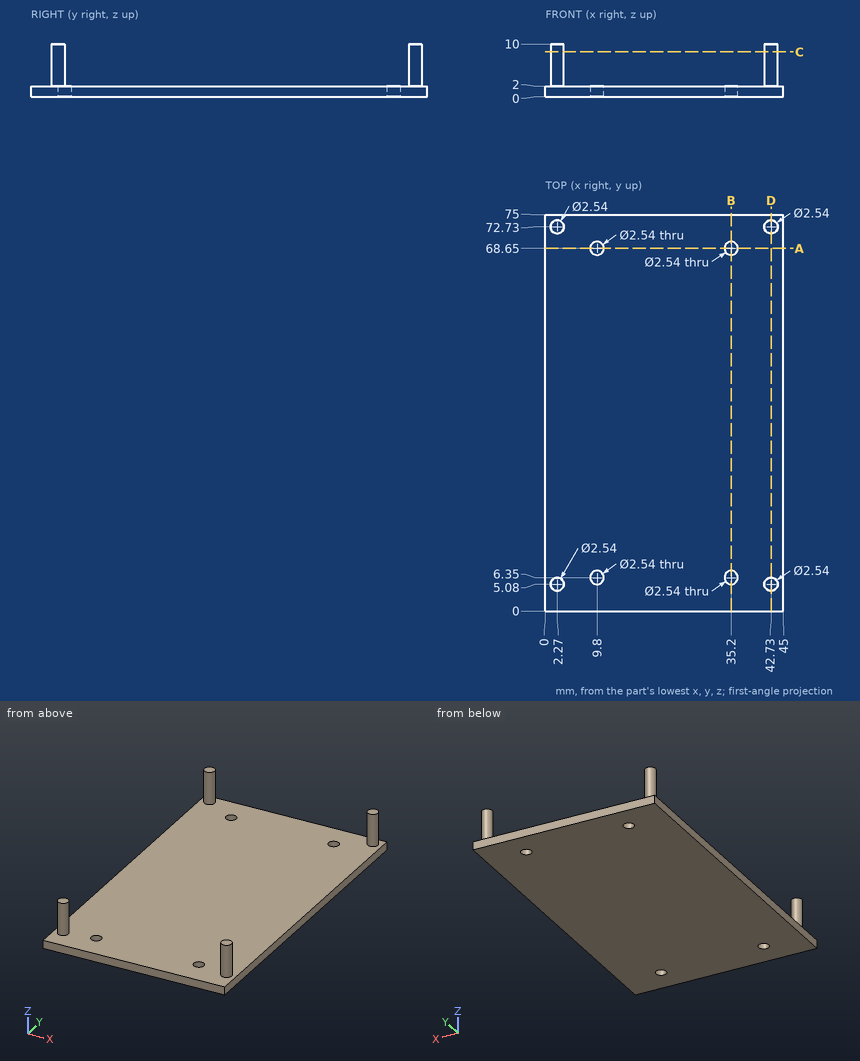
Geometry check sheet. Reference: drawing and pictorial views, mm from the part's lowest x, y, z. Give positions to 0.01 mm unless a question says otherwise; leave off trailing zeros. Order: outer loops, then holes, each group sorted by start corner. A loop starts at its lowest first (then second) coordinate and runs counter-clockwise, first axis right, second up. Notation, with made-up numbers: M 85,-39.5 L 135,-39.5 A7 cw 135,-35.5 Z; hole C 66,86 d6. An arc over 180 degrees is marked long. Answer as a JSON object with one key per item and string values. Group by question number.
1) Cross-section at D-D (x = 42.73). Enter the section's corners in (y, z), then the cut area to 3 significant figures.
2) Depth check by flat-ended pin: pin 1 Ø4 at (x, y) = (35.2, 68.65) entering from +Z. Enter the tip coordinate at first touch or a pass-through.
3) Cross-section at B-B (x = 35.2). Enter the section's corners in (y, z).
4) Scan lines: line 1 along X through (y, z) = (68.65, 0.85); line 2 along Z through (x, y) = (3, 44.5); line 3 along Y through (x, z) = (43.5, 7.5). Record each from-to range of solid material in increasing order. Write a range as [from, to].
5) Cross-section at A-A (y = 68.65). Enter the section's corners in (x, z).
6) Cross-section at C-C (z = 8.5). Enter the section's corners in (x, y).
Result sheet:
{
 "1": {"outline": "M 0,0 L 75,0 L 75,2 L 74,2 L 74,10 L 71.46,10 L 71.46,2 L 6.35,2 L 6.35,10 L 3.81,10 L 3.81,2 L 0,2 Z", "area": "191 mm2"},
 "2": {"pin 1": "stops at z = 2"},
 "3": {"outline": "M 0,0 L 5.08,0 L 5.08,2 L 0,2 Z; M 7.62,0 L 67.38,0 L 67.38,2 L 7.62,2 Z; M 69.92,0 L 75,0 L 75,2 L 69.92,2 Z"},
 "4": {"line 1": "x = [0, 8.53], [11.07, 33.93], [36.47, 45]", "line 2": "z = [0, 2]", "line 3": "y = [4.07, 6.09], [71.72, 73.74]"},
 "5": {"outline": "M 0,0 L 8.53,0 L 8.53,2 L 0,2 Z; M 11.07,0 L 33.93,0 L 33.93,2 L 11.07,2 Z; M 36.47,0 L 45,0 L 45,2 L 36.47,2 Z"},
 "6": {"outline": "C 2.27,5.08 d2.54; C 2.27,72.73 d2.54; C 42.73,5.08 d2.54; C 42.73,72.73 d2.54"}
}
